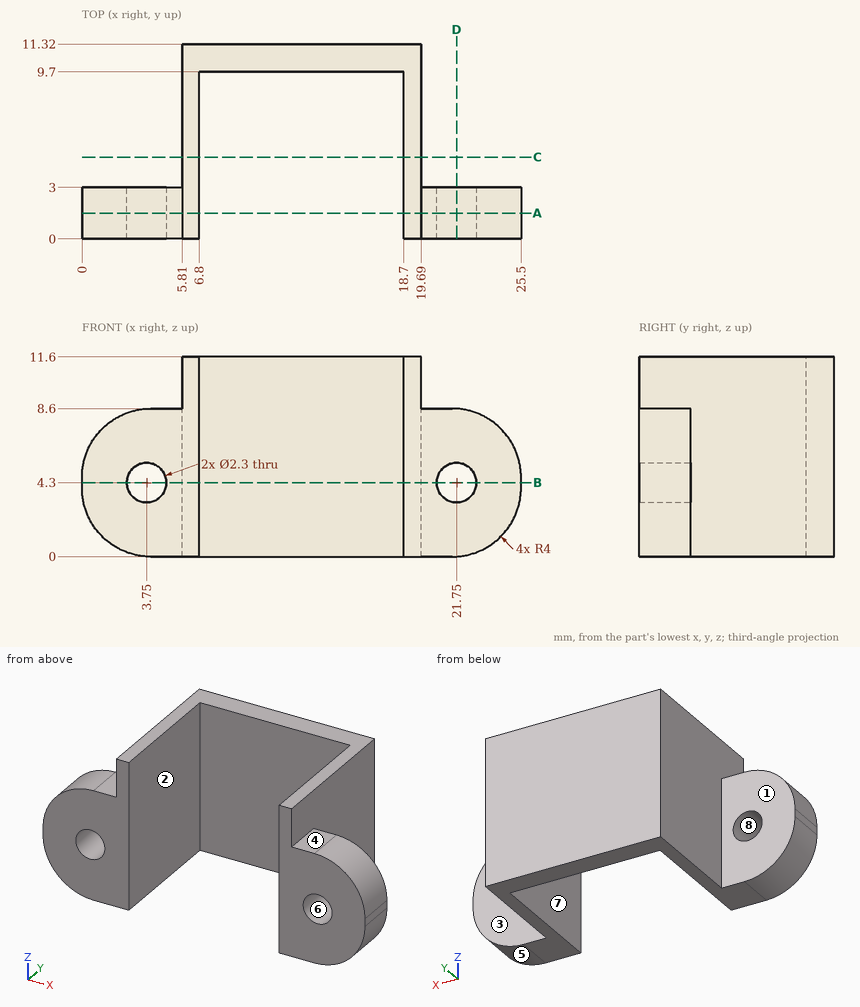
Check sheet for the drawn part. Datum: minimum x, y, z corner. Units: mm. A direction names the side the tool comes from. Give positions to 0.01 mm unless a question says otherwise; leave off trailing zeros. Order: outer loops, then holes, each group sorted by start corner. A loop starts at its lowest first (then second) coordinate and runs counter-clockwise, first axis right, second up.
1. Access from +Z, -Z, +X, -X, +Y, -Y to the whole of each face (thin tool, end or side, straight path). Record for the marked faces 1, 2, 3 and 4.
Completed:
face 1: +Z, -Z, -X, +Y
face 2: +Z, -Z, -Y
face 3: +Z, -Z, +X, +Y
face 4: +Z, +X, +Y, -Y
2. Sectioned sample at C-C (y = 4.75). Record the boundary of the cut face in (x, z).
Completed:
outline: (5.81, 0) - (6.8, 0) - (6.8, 11.6) - (5.81, 11.6) - close; (18.7, 0) - (19.69, 0) - (19.69, 11.6) - (18.7, 11.6) - close
3. Sectioned sample at D-D (x = 21.75). Record the boundary of the cut face in (y, z), then the cut area to 3 significant figures.
Completed:
outline: (0, 0.01) - (3, 0.01) - (3, 3.15) - (0, 3.15) - close; (0, 5.45) - (3, 5.45) - (3, 8.59) - (0, 8.59) - close
area: 18.9 mm2
4. Depth check by flat-ended pin: pin 1 (1.5 mm diameter, centred on x = 9.5, z = 8, fed in from -Y); pin 2 (3 mm diameter, centred on x = 1.5, z = 5, fed in from +Y); pin 3 (2.5 mm diameter, centred on x = 21.75, z = 4.3, fed in from -Y); pin 4 (0.9 mm diameter, centred on x = 4.5, y = 1.5, fed in from +Z). Enter the tip coordinate at first touch or a pass-through.
Completed:
pin 1: stops at y = 9.7
pin 2: stops at y = 3
pin 3: stops at y = 0
pin 4: stops at z = 8.6
5. Sectioned sample at B-B (z = 4.3). Record the boundary of the cut face in (x, y), then the cut area to 3 significant figures.
Completed:
outline: (0, 0) - (2.6, 0) - (2.6, 3) - (0, 3) - close; (4.9, 0) - (6.8, 0) - (6.8, 9.7) - (18.7, 9.7) - (18.7, 0) - (20.6, 0) - (20.6, 3) - (19.69, 3) - (19.69, 11.32) - (5.81, 11.32) - (5.81, 3) - (4.9, 3) - close; (22.9, 0) - (25.5, 0) - (25.5, 3) - (22.9, 3) - close
area: 62.8 mm2
6. Scan lines: line 1 (X direction, y = 1.85, z = 4.3); line 2 (X direction, y = 8.5, z = 6.5); line 3 (Y direction, x = 3, z = 0.75). Record each from-to range of solid material in increasing order.
Completed:
line 1: x = 0 to 2.6, 4.9 to 6.8, 18.7 to 20.6, 22.9 to 25.5
line 2: x = 5.81 to 6.8, 18.7 to 19.69
line 3: y = 0 to 3
7. Draft check along Z on the marked faces 5, 6, 7 and 8. Enter one of: pulls with the +Z half, pulls with the -Z half, needs draft (parallel to the pull), parting line crosses it, or undercut.
Completed:
face 5: pulls with the -Z half
face 6: undercut
face 7: needs draft
face 8: undercut
8. Sectioned sample at A-A (y = 1.5). Record the boundary of the cut face in (x, z), then the cut area to 3 significant figures.
Completed:
outline: (0, 4) arc R4 ccw to (4, 0) - (6.8, 0) - (6.8, 11.6) - (5.81, 11.6) - (5.81, 8.6) - (4, 8.6) arc R4 ccw to (0, 4.6) - close; (18.7, 0) - (21.5, 0) arc R4 ccw to (25.5, 4) - (25.5, 4.6) arc R4 ccw to (21.5, 8.6) - (19.69, 8.6) - (19.69, 11.6) - (18.7, 11.6) - close; hole circle Ø2.3 at (3.75, 4.3); hole circle Ø2.3 at (21.75, 4.3)
area: 101 mm2
